Read the model definition and answer for the solid it produces. Units are mm, in the model's axes. A direction names the side the tool comes from. Give positions to 0.01 mm unless a question says otherwise; leave off trailing zeros. Order: outer loops, then holes, each group sorted by start corner. A loop starts at its lowest first (then second) coordinate and runs counter-clockwise, first axis right, second up. Notation, with made-up numbers: (-25.5, 86.25) - (-6.5, 86.25) arc R19 ccw to (-6.5, 99.25) - close; hole circle Ø5 at (-24.75, 67.25). An arc over 180 degrees is marked (long way). Write item = value, one per line.
```python
from build123d import *

# Parameters (mm, degrees)
SKETCH1_R                   = 15.875
SKETCH1_R_2                 = 1.778
BOSS_EXTRUDE1_DEPTH         = 6.35
F_1_4_CLEARANCE_HOLE2_D     = 6.7564
F_1_4_CLEARANCE_HOLE2_DEPTH = 6.35
FILLET1_R                   = 6.35


with BuildPart() as part:
    # Sketch1 → Boss-Extrude1 (new body)
    with BuildSketch(Plane(origin=(0, 0, 0), x_dir=(1, 0, 0), z_dir=(0, 1, 0))):
        with BuildLine():
            Line((-113.03, 25.4), (-113.03, -25.4))
            Line((-113.03, -25.4), (77.47, -25.4))
            ThreePointArc((77.47, -25.4), (81.960128061, -23.540128061), (83.82, -19.05))
            Line((83.82, -19.05), (83.82, 19.05))
            ThreePointArc((83.82, 19.05), (81.960128061, 23.540128061), (77.47, 25.4))
            Line((77.47, 25.4), (-113.03, 25.4))
        make_face()
        with Locations((12.7, 0)):
            Circle(SKETCH1_R, mode=Mode.SUBTRACT)
        with Locations((64.008, 0)):
            Circle(SKETCH1_R, mode=Mode.SUBTRACT)
        with Locations((0, 18.288)):
            Circle(SKETCH1_R_2, mode=Mode.SUBTRACT)
        with Locations((25.4, 18.288)):
            Circle(SKETCH1_R_2, mode=Mode.SUBTRACT)
        with Locations((51.308, 18.288)):
            Circle(SKETCH1_R_2, mode=Mode.SUBTRACT)
        with Locations((76.708, 18.288)):
            Circle(SKETCH1_R_2, mode=Mode.SUBTRACT)
        with Locations((0, -18.288)):
            Circle(SKETCH1_R_2, mode=Mode.SUBTRACT)
        with Locations((25.4, -18.288)):
            Circle(SKETCH1_R_2, mode=Mode.SUBTRACT)
        with Locations((51.308, -18.288)):
            Circle(SKETCH1_R_2, mode=Mode.SUBTRACT)
        with Locations((76.708, -18.288)):
            Circle(SKETCH1_R_2, mode=Mode.SUBTRACT)
        with BuildLine():
            Line((-30.48, 17.78), (-45.72, 17.78))
            ThreePointArc((-45.72, 17.78), (-63.5, 0), (-45.72, -17.78))
            Line((-45.72, -17.78), (-30.48, -17.78))
            ThreePointArc((-30.48, -17.78), (-12.7, 0), (-30.48, 17.78))
        make_face(mode=Mode.SUBTRACT)
    extrude(amount=BOSS_EXTRUDE1_DEPTH)

    # 1/4 Clearance Hole2
    with Locations(Plane(origin=(0, 6.35, 0), x_dir=(1, 0, 0), z_dir=(0, 1, 0))):
        with Locations((-103.505, 15.875), (-69.85, 15.875), (-69.85, -15.875), (-103.505, -15.875)):
            Hole(F_1_4_CLEARANCE_HOLE2_D / 2, depth=F_1_4_CLEARANCE_HOLE2_DEPTH)

    # Fillet1
    fillet1_edges = [part.edges().sort_by_distance(p)[0] for p in [
        (-113.03, 3.175, 25.4),
        (-113.03, 3.175, -25.4),
    ]]
    fillet(fillet1_edges, radius=FILLET1_R)


solid = part.part
```
1. Section C-C (x = -69.85) is taken. Determine the outline of the cut face in (y, z), and give its area (3 significant figures).
Recorded:
outline = (0, -25.4) - (6.35, -25.4) - (6.35, -19.25) - (0, -19.25) - close; (0, -12.5) - (6.35, -12.5) - (6.35, 12.5) - (0, 12.5) - close; (0, 19.25) - (6.35, 19.25) - (6.35, 25.4) - (0, 25.4) - close
area = 237 mm^2
2. Section D-D (y = 3.25) is taken. Count the separate pieces of the cut face and the enclosed holes in it, and give its area (3 significant figures).
Recorded:
separate_pieces = 1
enclosed_holes = 15
area = 6,620 mm^2
3. A flat-ended cylindrical pin translates along its axis: pin 1 (4.5 mm diameter, centred on x = 51.308, z = -18.288, fed in from +Y). Find the tip coordinate at first contact, or state that the pin passes through.
Recorded:
pin_1 = 6.35
4. Determine the mould class of faces 1 (the face through (-38, 3, 17.78)), 2 (the face through (-111.22, 3.22, 23.49)), 3 (the face through (82, 3.1, -23.5)) for opening direction X: +X half, -X half, draft (parallel to the pull), parting line (faces both ways), or undercut.
Recorded:
face_1 = undercut
face_2 = -X half
face_3 = +X half
5. Section B-B (z = 0) is taken. Determine the outline of the cut face in (x, y) (3 decimals), and give its area (3 significant figures).
Recorded:
outline = (-113.03, 0) - (-63.5, 0) - (-63.5, 6.35) - (-113.03, 6.35) - close; (-12.7, 0) - (-3.175, 0) - (-3.175, 6.35) - (-12.7, 6.35) - close; (28.575, 0) - (48.133, 0) - (48.133, 6.35) - (28.575, 6.35) - close; (79.883, 0) - (83.82, 0) - (83.82, 6.35) - (79.883, 6.35) - close
area = 524 mm^2
6. Straight lines are drawn through the part: L1, parallel to X at y = 2.5, z = -1; L2, parallel to X at y = 2, z = 14; L3, parallel to Z at x = -34.5, y = 0.5. For each, find the intervals that lie inside material, in ascending order. Write a range as [from, to].
Recorded:
L1 = [-113.03, -63.47], [-12.73, -3.14], [28.54, 48.16], [79.85, 83.82]
L2 = [-113.03, -106.32], [-100.69, -72.66], [-67.04, -56.68], [-19.52, 5.22], [20.18, 56.52], [71.49, 83.82]
L3 = [-25.4, -17.78], [17.78, 25.4]
7. Section A-A (x = 12.7) is taken. Determine the outline of the cut face in (y, z) (3 decimals), and give its area (3 significant figures).
Recorded:
outline = (0, -25.4) - (6.35, -25.4) - (6.35, -15.875) - (0, -15.875) - close; (0, 15.875) - (6.35, 15.875) - (6.35, 25.4) - (0, 25.4) - close
area = 121 mm^2
8. For faces 4 (the face through (-38, 3, -17.78)), 5 (the face through (-16, 3, 25.4)), determine the directions among +Z, -Z, +X, -X, +Y, -Y from which every point of the face is accessible in a straight line to the end or side of a thin tool.
Recorded:
face_4 = +Y, -Y
face_5 = +Z, +X, -X, +Y, -Y
